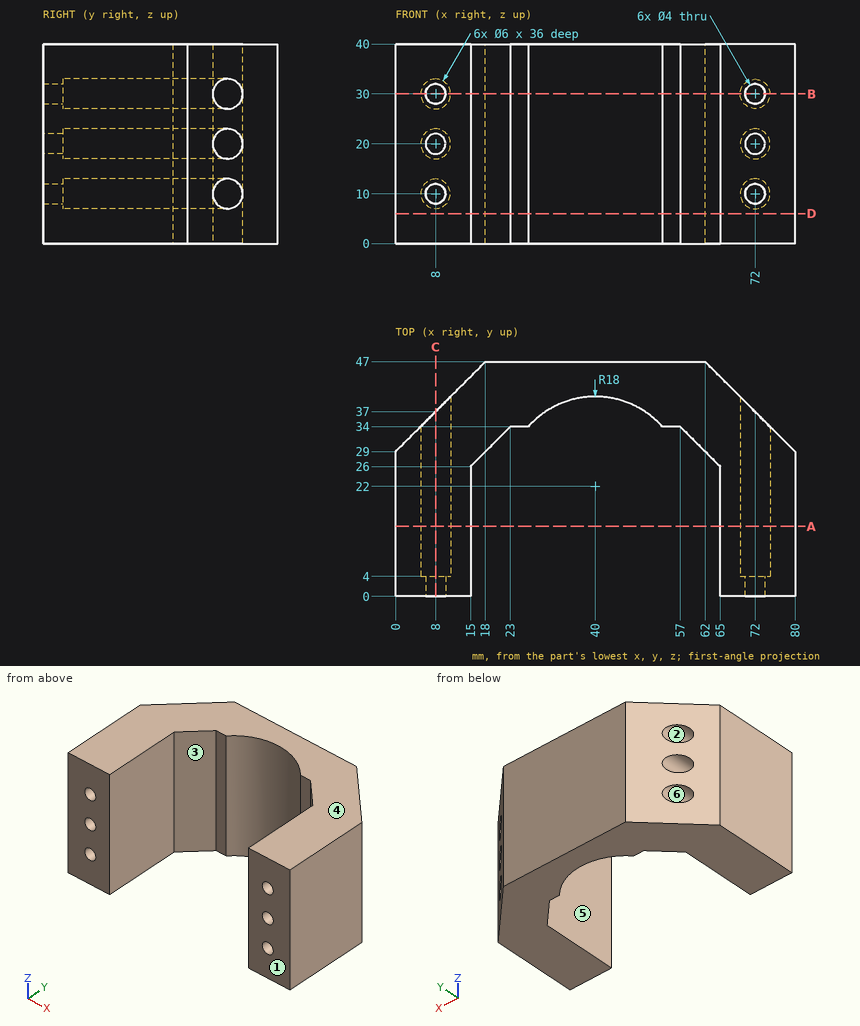
Part print with two shaded views. Sizes in mm from the minimum x, y, z corner. A direction names the side the tool comes from. Coordinates: 2 decimals unless noted, no trailing zeros. Write each loop counter-clockwise with the first axis right and the second up, starting at its lowest first coordinate (ties: lowest second). Pieces come first, ordered by that corner, then holes. Notation, with made-up numbers: M 13.25,53.25 L 26.25,53.25 A31 ccw 26.25,82.25 Z; hole C 87.25,11 d3. An arc over 180 degrees is marked long. Return JSON: item names as keys, results as strings.
Item 1: Drop flat-ended pins along their axis: pin 1 Ø1.1 at (x, z) = (54.5, 17.5) entering from -Y; pin 2 Ø3.5 at (x, z) = (72, 10) entering from -Y; pin 3 Ø1 at (y, z) = (39.5, 19) entering from +X; pin 4 Ø5 at (x, z) = (8, 10) entering from +Y. Give the stop position or say it passes through.
Findings below:
{"pin 1": "stops at y = 34", "pin 2": "passes through", "pin 3": "stops at x = 69.4", "pin 4": "stops at y = 4"}
Item 2: Slice it at B-B, the plane z = 30. State how many separate pieces and enclosed holes the cut face has, and give its area (3 significant figures).
Findings below:
{"separate pieces": "3", "enclosed holes": "0", "area": "1,260 mm2"}
Item 3: Probe line 1 (X direction, y = 2, z = 10); line 2 (Z direction, x = 8, y = 1.4); line 3 (X direction, y = 18, z = 10). List the from-to ranges inside material, lowest first. Write a range as from..to.
Findings below:
{"line 1": "x = 0..6, 10..15, 65..70, 74..80", "line 2": "z = 0..8, 12..18, 22..28, 32..40", "line 3": "x = 0..5, 11..15, 65..69, 75..80"}
Item 4: Which spindle directions (+Z, -Z, +X, -X, +Y, -Y) get a long thin tool onto all of the face, cutting with end or side? Do the marked faces 1, 2 and 3. Say none if no direction does.
Findings below:
{"face 1": "+Z, -Z, +X, -X, -Y", "face 2": "+Y", "face 3": "+Z, -Z, -Y"}
Item 5: Slice it at C-C, the plane x = 8. Write the cut outline in (y, z).
Findings below:
{"outline": "M 0,0 L 37,0 L 37,7 L 4,7 L 4,8 L 0,8 Z; M 0,12 L 4,12 L 4,13 L 37,13 L 37,17 L 4,17 L 4,18 L 0,18 Z; M 0,22 L 4,22 L 4,23 L 37,23 L 37,27 L 4,27 L 4,28 L 0,28 Z; M 0,32 L 4,32 L 4,33 L 37,33 L 37,40 L 0,40 Z"}
Item 6: Slice it at A-A, the plane y = 14. Write the cut outline in (x, z), and give its area (3 significant figures).
Findings below:
{"outline": "M 0,0 L 15,0 L 15,40 L 0,40 Z; M 65,0 L 80,0 L 80,40 L 65,40 Z; hole C 8,10 d6; hole C 8,20 d6; hole C 8,30 d6; hole C 72,10 d6; hole C 72,20 d6; hole C 72,30 d6", "area": "1,030 mm2"}
Item 7: Slice it at D-D, the plane z = 6. Write the cut outline in (x, y).
Findings below:
{"outline": "M 0,0 L 15,0 L 15,26 L 23,34 L 26.58,34 A18 cw 53.42,34 L 57,34 L 65,26 L 65,0 L 80,0 L 80,29 L 62,47 L 18,47 L 0,29 Z"}
Item 8: Two-plate mould, pull along Z, no slides. Class the marked faces 4, 5 and 6: +Z half, -Z half, draft (parallel to the pull), parting line (faces both ways), or undercut.
Findings below:
{"face 4": "+Z half", "face 5": "draft", "face 6": "undercut"}
